The model under review builds one solid part; all positions refer to its coordinate system, in mm. Face numbers are marked on the shaded views. A direction names the side the tool comes from. Give positions to 0.01 mm unless a question says otherwise; leave off trailing zeros. Loops run counter-clockwise (first coordinate to the right, second up) from the corner with the lowest first, then second, coordinate; pieces in that order, holes last. Notation, with made-up numbers: M 31,35 L 60,35 A10 ccw 60,39 Z; hole C 15,29 d6. An arc over 180 degrees is marked long. Return JSON: item names as keys, results as strings.
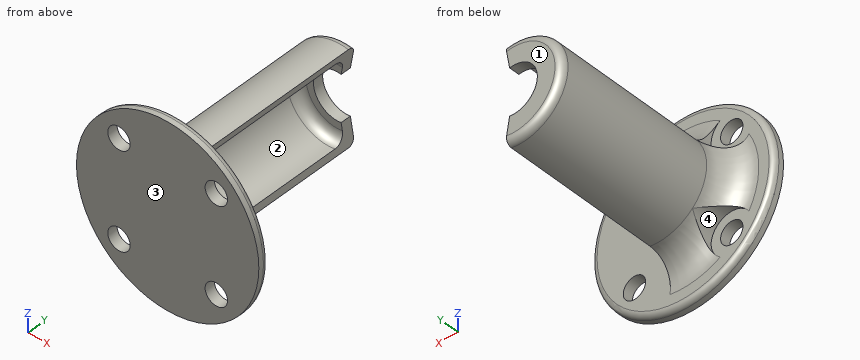
Autodesk Inventor part; units mm, degrees
ref_plane "YZ Plane" through (0, 0, 0) normal (1, 0, 0) x (0, 1, 0)
ref_plane "XZ Plane" through (0, 0, 0) normal (0, 1, 0) x (-1, 0, 0)
ref_plane "XY Plane" through (0, 0, 0) normal (0, 0, 1) x (1, 0, 0)
sketch "Sketch1" plane through (0, 0, 0) normal (0, 1, 0) x (-1, 0, 0)
  circle A0 centre (0, 0) radius 26.5
  circle A1 centre (-14.1421, 14.1421) radius 3.25
  circle A2 centre (-14.1421, -14.1421) radius 3.25
  circle A3 centre (14.1421, -14.1421) radius 3.25
  circle A4 centre (14.1421, 14.1421) radius 3.25
  line L0 (0, 0) -> (0, 26.5) construction
  line L1 (0, 0) -> (-18.7383, 18.7383) construction
  dimension "d0" = 53
  dimension "d1" = 6.5
  dimension "d2" = 20
  dimension "d5" = 360
  dimension "d9" = 45
extrude "Extrusion1" add sketch "Sketch1" along normal blind 3
sketch "Sketch2" plane through (0, 0, 0) normal (0, 0, 1) x (1, 0, 0)
  line L0 (26.5, 3) -> (-26.5, 3)
  line L1 (-12, 3) -> (-14, 3)
  line L2 (-14, 3) -> (-14, 58)
  line L3 (-14, 58) -> (-12, 58)
  line L4 (-12, 58) -> (-12, 3)
  line L5 (-14, 58) -> (-6.85, 58)
  line L6 (-6.85, 58) -> (-6.85, 55)
  line L7 (-6.85, 55) -> (-14, 55)
  line L8 (-14, 55) -> (-14, 58)
  line L9 (0, -11.6) -> (0, 69.6)
  point P0 (0, 0)
  point P1 (-12, 55)
  dimension "d10" = 12
  dimension "d11" = 6.85
  dimension "d12" = 2
  dimension "d13" = 55
  dimension "d14" = 3
revolve "Revolution1" add sketch "Sketch2" angle 200 mid plane about axis through (0, -10, 0) along (0, 1, 0)
fillet "Fillet1" radius 8 1 edges at (-14, 3, 0)
fillet "Fillet1" radius 3 1 edges at (-12, 55, 0)
fillet "Fillet1" radius 3 1 edges at (-12, 3, 0)
fillet "Fillet1" radius 2 1 edges at (-14, 58, 0)
fillet "Fillet1" radius 1.5 1 edges at (26.5, 3, 0)
sketch "Sketch3" plane through (0, 3, 0) normal (0, 1, 0) x (1, 0, 0)
  circle A0 centre (14.1421, 14.1421) radius 3.25
  circle A1 centre (14.1421, 14.1421) radius 6
  circle A2 centre (-14.1421, 14.1421) radius 6
  circle A3 centre (-14.1421, -14.1421) radius 6
  circle A4 centre (14.1421, -14.1421) radius 6
  arc A5 (2.4311, 13.7873) -> (2.4311, -13.7873) centre (0, 0) ccw
  dimension "d23" = 360
  dimension "d27" = 12
extrude "Extrusion2" cut sketch "Sketch3" along normal blind 8 contours A0 | A1 | A2 | A3 | A4
properties part number "_3DPrint"
1) Consider section A-A on x = 0. Write out the cut boundary in (y, z).
From the geometry:
{"outline": "M 0,-26.5 L 1.5,-26.5 A1.5 ccw 3,-25 L 3,-22 A8 cw 11,-14 L 56,-14 A2 ccw 58,-12 L 58,-6.85 L 55,-6.85 L 55,-9 A3 cw 52,-12 L 6,-12 A3 cw 3,-9 L 3,9 A3 cw 6,12 L 52,12 A3 cw 55,9 L 55,6.85 L 58,6.85 L 58,12 A2 ccw 56,14 L 11,14 A8 cw 3,22 L 3,25 A1.5 ccw 1.5,26.5 L 0,26.5 Z"}
2) The part is to be moulded in two halves that separate along X. For the marked faces 1 and 2, say which applies: released by +X, released by -X, zero draft, split by the parting line, or undercut.
From the geometry:
{"face 1": "zero draft", "face 2": "undercut"}
3) Consider section D-D on y = 32.5. Write out the cut boundary in (x, z), then the cut area to 3 significant figures.
From the geometry:
{"outline": "M 2.08,-11.82 A12 cw long 2.08,11.82 L 2.43,13.79 A14 ccw long 2.43,-13.79 Z", "area": "90.8 mm²"}
4) Consider section C-C on x = 16. Count the separate pieces of the cut face and the enclosed holes in it, then the cut area to 3 significant figures.
From the geometry:
{"separate pieces": "3", "enclosed holes": "0", "area": "93.5 mm²"}
5) Insertion check: pin 1 (10 mm diameter, centred on x = 1, y = 14, fed in from -Z); pin 2 (3 mm diameter, centred on x = 18, z = 15, fed in from -Y); pin 3 (3 mm diameter, centred on x = -6.5, y = 50.5, fed in from +Z); pin 4 (12 mm diameter, centred on y = 27.5, z = -4, fed in from +X). Each pin has a flat end and moves straight along its axis. Give the tip position at first contact, or say it passes through.
From the geometry:
{"pin 1": "z = -14.24", "pin 2": "y = 0", "pin 3": "z = 13.08", "pin 4": "x = -6.63"}
6) Wall thickness on L1, parallel to Y at x = 0.5, z = -9; L2, parallel to Z at x = 0, y = 35; L3, parallel to Y at x = 12, z = -3.5: over which ranges is each line inside the solid? List them lowest first. Write a range as from..to.
From the geometry:
{"L1": "0..3, 55..58", "L2": "-14..-12, 12..14", "L3": "0..3"}
7) Consider section B-B on z = 0. Write out the cut boundary in (x, y), then the cut area to 3 significant figures.
From the geometry:
{"outline": "M -26.5,0 L 26.5,0 L 26.5,1.5 A1.5 ccw 25,3 L -9,3 A3 cw -12,6 L -12,52 A3 cw -9,55 L -6.85,55 L -6.85,58 L -12,58 A2 ccw -14,56 L -14,11 A8 cw -22,3 L -25,3 A1.5 ccw -26.5,1.5 Z", "area": "300 mm²"}
8) Tool access review of the marked faces 3 and 4: name each direction out of +Z, -Z, +X, -X, +Y, -Y from which nothing blocks a thin tool from reaching the whole face with its end or side.
From the geometry:
{"face 3": "+Z, -Z, +X, -X, -Y", "face 4": "+Y"}
